Model file for the job. Use its own axes, mm. Face numbers are marked on the shaded views. A direction names the side the tool comes from. Give positions to 0.01 mm unless a question says otherwise; leave off trailing zeros. Loops run counter-clockwise (first coordinate to the right, second up) from the corner with the lowest first, then second, coordinate; pieces in that order, holes last. Notation, with made-up numbers: (13, -18) - (28, -18) arc R27 cw to (28, 17) - close; hole circle Ø10 at (83, 32). An arc over 180 degrees is marked (long way). Use a Markdown table: item, result.
Autodesk Inventor part; units mm, degrees
ref_plane "YZ Plane" through (0, 0, 0) normal (1, 0, 0) x (0, 1, 0)
ref_plane "XZ Plane" through (0, 0, 0) normal (0, 1, 0) x (-1, 0, 0)
ref_plane "XY Plane" through (0, 0, 0) normal (0, 0, 1) x (1, 0, 0)
sketch "Sketch1" plane through (0, 0, 0) normal (0, 1, 0) x (-1, 0, 0)
  line L0 (0, 0) -> (12.7, 0)
  line L1 (12.7, 0) -> (12.7, -38.1)
  line L2 (12.7, -38.1) -> (0, -38.1)
  line L3 (0, -38.1) -> (0, 0)
  line L4 (6.35, 0) -> (6.35, -6.35)
  circle A0 centre (6.35, -6.35) radius 2.1082
  line L5 (6.35, -6.35) -> (6.35, -19.05)
  line L6 (6.35, -19.05) -> (6.35, -31.75)
  circle A1 centre (6.35, -19.05) radius 2.1082
  circle A2 centre (6.35, -31.75) radius 2.1082
  dimension "d0" = 12.7
  dimension "d1" = 38.1
  dimension "d2" = 6.35
  dimension "d3" = 4.2164
  dimension "d4" = 12.7
  dimension "d5" = 12.7
  dimension "d6" = 4.2164
  dimension "d7" = 4.2164
extrude "Extrusion1" add sketch "Sketch1" along normal blind 19.1516
sketch "Sketch2" plane through (0, 0, 0) normal (0, -1, 0) x (1, 0, 0)
  circle A0 centre (-6.35, -19.05) radius 2.1082
  circle A1 centre (-6.35, -19.05) radius 5.08
  point P0 (0, 0)
  dimension "d11" = 10.16
extrude "Extrusion2" cut sketch "Sketch2" against normal blind 6.35
sketch "Sketch3" plane through (0, 0, 0) normal (0, -1, 0) x (1, 0, 0)
  line L0 (-12.7, -38.1) -> (-12.7, 0)
  line L1 (-12.7, 0) -> (-12.7, -10.795)
  line L2 (-12.7, -10.795) -> (0, -10.795)
  line L3 (0, 0) -> (0, -38.1)
  line L4 (0, 0) -> (-12.7, 0)
  point P0 (0, -3.175)
  dimension "d15" = 10.795
extrude "Extrusion3" add sketch "Sketch3" along normal blind 1.5875
fillet "Fillet3" radius 3.175 1 edges at (0, 8.782, 0)
sketch "Sketch4" plane through (-6.35, 0, -6.35) normal (0, 1, 0) x (1, 0, 0)
  circle A0 centre (0, 0) radius 2.1082
  point P0 (6.35, -6.35)
extrude "Extrusion4" cut sketch "Sketch4" against normal blind 3.175
fillet "Fillet4" radius 3.175 1 edges at (0, 9.5758, -38.1)
properties part number "inner wing mount"
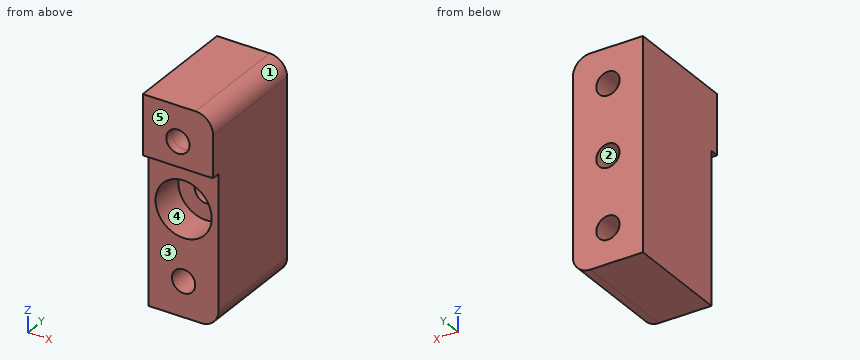
(1) Drill centre lines: probe 1 along Z at (x, y) = (-6.35, 4); probe 2 along Z at (x, y) = (-6.35, 14); probe 3 along Z at (x, y) = (-6.35, -0.75) (3 decimals). Where is each one in solid material? Low to high. Write a range as [from, to].
Computed:
| item | result |
|---|---|
| probe 1 | [-38.1, -33.86], [-29.64, -24.13], [-13.97, -8.46], [-4.24, 0] |
| probe 2 | [-38.1, -33.86], [-29.64, -21.16], [-16.94, -8.46], [-4.24, 0] |
| probe 3 | [-10.795, -8.458], [-4.242, 0] |
(2) Slice it at A-A, the plane z = -19.05. Write the cut outline in (x, y).
Computed:
| item | result |
|---|---|
| outline | (-12.7, 0) - (-11.43, 0) - (-11.43, 6.35) - (-8.46, 6.35) - (-8.46, 19.15) - (-12.7, 19.15) - close; (-4.24, 6.35) - (-1.27, 6.35) - (-1.27, 0) - (0, 0) - (0, 19.15) - (-4.24, 19.15) - close |
(3) 3-axis set-ups, long thin cutter, end or side, ignore diameter. For the marked faces 4 and 5: which of +Z, -Z, +X, -X, +Y, -Y reach the whole face in a straight line?
Computed:
| item | result |
|---|---|
| face 4 | -Y |
| face 5 | +Z, -Z, +X, -X, -Y |
(4) Pin check, flat tips, straight feed: P1, Ø1.7, axis at x = -8.5, y = -1, coming from the -Z side (3 decimals); P2, Ø4, axis at x = -5.5, z = -20, coming from the -Y side; P3, Ø5, axis at x = -5.5, z = -27, coming from the -Y side. Stop position of each tip, or through.
Computed:
| item | result |
|---|---|
| P1 | z = -10.795 |
| P2 | y = 6.35 |
| P3 | y = 0 |
(5) Slice it at C-C, the plane x = -8. Count the separate pieces of the cut face and the enclosed holes in it, plus the area to 3 significant figures.
Computed:
| item | result |
|---|---|
| separate pieces | 4 |
| enclosed holes | 0 |
| area | 548 mm² |
(6) Slice it at D-D, the plane z = -31.75. Write the cut outline in (x, y), plus the area to 3 significant figures.
Computed:
| item | result |
|---|---|
| outline | (-12.7, 0) - (-8.46, 0) - (-8.46, 19.15) - (-12.7, 19.15) - close; (-4.24, 0) - (0, 0) - (0, 19.15) - (-4.24, 19.15) - close |
| area | 162 mm² |
(7) Mould opens along Z. For the marked faces 1, 2 and 3 say: pulls with the +Z half, pulls with the -Z half, needs draft (parallel to the pull), parting line crosses it, or undercut.
Computed:
| item | result |
|---|---|
| face 1 | pulls with the +Z half |
| face 2 | undercut |
| face 3 | needs draft |
(8) Slice it at B-B, the plane y = 5. Write the cut outline in (x, z) (3 decimals).
Computed:
| item | result |
|---|---|
| outline | (-12.7, -38.1) - (-3.175, -38.1) arc R3.175 ccw to (0, -34.925) - (0, -3.175) arc R3.175 ccw to (-3.175, 0) - (-12.7, 0) - close; hole circle Ø10.16 at (-6.35, -19.05); hole circle Ø4.216 at (-6.35, -31.75); hole circle Ø4.216 at (-6.35, -6.35) |
